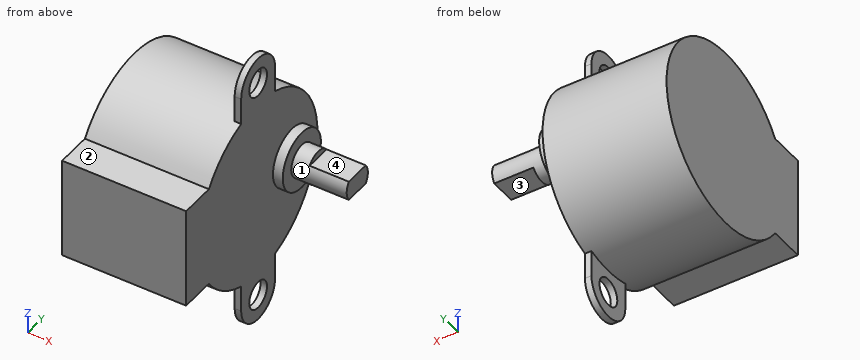
Autodesk Inventor part; units mm, degrees
ref_plane "YZ Plane" through (0, 0, 0) normal (1, 0, 0) x (0, 1, 0)
ref_plane "XZ Plane" through (0, 0, 0) normal (0, 1, 0) x (-1, 0, 0)
ref_plane "XY Plane" through (0, 0, 0) normal (0, 0, 1) x (1, 0, 0)
sketch "Boceto1" plane through (0, 0, 0) normal (1, 0, 0) x (0, 1, 0)
  circle A0 centre (0, 0) radius 14
  dimension "d0" = 28
extrude "Extrusión1" add sketch "Boceto1" along normal blind 19
sketch "Boceto2" plane through (19, 0, 0) normal (1, 0, 0) x (0, 0, -1)
  line L0 (0, 0) -> (0, 8)
  circle A0 centre (0, 8) radius 4.5
  dimension "d3" = 8
  dimension "d4" = 9
extrude "Extrusión2" add sketch "Boceto2" along normal blind 1.5
sketch "Boceto3" plane through (20.5, 8, 0) normal (1, 0, 0) x (0, 0, -1)
  circle A0 centre (0, 0) radius 2.5
  point P0 (0, -8)
  dimension "d7" = 5
extrude "Extrusión3" add sketch "Boceto3" along normal blind 2.5
sketch "Boceto4" plane through (23, 8, 0) normal (1, 0, 0) x (0, 0, -1)
  line L0 (0, 0) -> (-1.5, 0)
  line L1 (-1.5, 0) -> (-1.5, 3)
  line L2 (-1.5, 3) -> (-1.5, -3)
  line L3 (-1.5, -3) -> (1.5, -3)
  line L4 (1.5, -3) -> (1.5, 2.8642)
  circle A0 centre (0, 0) radius 2.5
  point P0 (0, -8)
  point P1 (1.5, 2)
  point P2 (-1.5, 2)
  point P3 (-1.5, -2)
  point P4 (1.5, -2)
  dimension "d10" = 1.5
  dimension "d11" = 3
extrude "Extrusión4" add sketch "Boceto4" along normal blind 6 contours L1 A0 L4 L2
sketch "Boceto5" plane through (19, 0, 0) normal (1, 0, 0) x (0, 0, -1)
  line L0 (0, 0) -> (17.5, 0)
  circle A0 centre (17.5, 0) radius 2.1
  arc A1 (17.5, -4) -> (17.5, 4) centre (17.5, 0) ccw
  line L1 (17.5, 4) -> (-17.5, 4)
  line L2 (0, 0) -> (0, 18)
  line L3 (-15.4, 0) -> (-17.5, 0)
  circle A2 centre (-17.5, 0) radius 2.1
  arc A3 (-17.5, 4) -> (-17.5, -4) centre (-17.5, 0) ccw
  line L4 (17.5, -4) -> (-17.5, -4)
  dimension "d18" = 4.2
  dimension "d14" = 17.5
  dimension "d15" = 4.2
  dimension "d16" = 8
  dimension "d17" = 17.5
  dimension "d19" = 8
extrude "Extrusión5" add sketch "Boceto5" against normal blind 1
sketch "Boceto6" plane through (19, 0, 0) normal (1, 0, 0) x (0, 0, -1)
  line L0 (0, 0) -> (0, -17)
  line L1 (0, -17) -> (7.8, -17)
  line L2 (0, -17) -> (-7.8, -17)
  line L3 (-7.8, -17) -> (7.8, -17)
  line L4 (7.8, -17) -> (7.8, -6)
  line L5 (7.8, -6) -> (-7.8, -6)
  line L6 (-7.8, -6) -> (-7.8, -17)
  dimension "d22" = 17
  dimension "d23" = 7.8
  dimension "d25" = 7.8
extrude "Extrusión6" add sketch "Boceto6" against normal blind 19
properties part number "MOTOR"
Design review of the part built by this model. Coordinates are the model's own, in mm. Face numbers are marked on the shaded views. A direction names the side the tool comes from. Give positions to 0.01 mm unless a question says otherwise; leave off trailing zeros. Write each loop counter-clockwise with the first axis right and the second up, starting at its lowest first coordinate (ties: lowest second). Pieces come first, ordered by that corner, then holes. Notation, with made-up numbers: M -10.5,11.5 L 46.5,11.5 A21 cw 46.5,16.5 Z; hole C 10,2.5 d2. An arc over 180 degrees is marked long. Return JSON: item names as keys, results as strings. Group by question number.
Item 1: Tool access review of the marked faces 1, 2, 3 and 4: name each direction out of +Z, -Z, +X, -X, +Y, -Y from which nothing blocks a thin tool from reaching the whole face with its end or side.
Item 2: Take a section at B-B (z = 0). Give the boundary of the cut face in (x, y).
Item 3: Take a section at A-A (y = 0). Give the boundary of the cut face in (x, z), plus the area to 3 significant figures.
Item 4: Take a section at C-C (x = 17.25). Give the boundary of the cut face in (y, z), plus the area to 3 significant figures.
Item 5: Wall thickness on line 1 along Y through (x, z) = (18.2, 17.5); line 2 along X through (y, z) = (-3, 10); line 3 along Z through (x, y) = (1.5, -13.5): over which ranges is each line inside the solid? List them lowest first.
Item 6: Take a section at D-D (z = -16). Give the boundary of the cut face in (x, y).
Item 7: Clearance check with flat-ended pins moving along their axes: pin 1 Ø6 at (x, y) = (13, 8.5) entering from +Z; pin 2 Ø6.5 at (y, z) = (0, -17.5) entering from +X; pin 3 Ø5 at (x, y) = (14, -11) entering from -Z; pin 4 Ø1.1 at (y, z) = (7.5, -2) entering from +X. State where each tip first meets the part, or that it passes through.
Return value:
{
 "1": {"face 1": "+X", "face 2": "+Z, +X, -X, -Y", "face 3": "-Z, +X, +Y, -Y", "face 4": "+Z, +X, +Y, -Y"},
 "2": {"outline": "M 0,-17 L 19,-17 L 19,3.5 L 20.5,3.5 L 20.5,5.5 L 29,5.5 L 29,10.5 L 20.5,10.5 L 20.5,12.5 L 19,12.5 L 19,14 L 0,14 Z"},
 "3": {"outline": "M 0,-14 L 18,-14 L 18,-15.4 L 19,-15.4 L 19,15.4 L 18,15.4 L 18,14 L 0,14 Z; M 18,-21.5 L 19,-21.5 L 19,-19.6 L 18,-19.6 Z; M 18,19.6 L 19,19.6 L 19,21.5 L 18,21.5 Z", "area": "539 mm2"},
 "4": {"outline": "M -17,-7.8 L -11.63,-7.8 A14 ccw long -11.63,7.8 L -17,7.8 Z", "area": "674 mm2"},
 "5": {"line 1": "y = -4 to -2.1, 2.1 to 4", "line 2": "x = 0 to 19", "line 3": "z = -7.8 to 7.8"},
 "6": {"outline": "M 18,-4 L 19,-4 L 19,-1.47 L 18,-1.47 Z; M 18,1.47 L 19,1.47 L 19,4 L 18,4 Z"},
 "7": {"pin 1": "stops at z = 12.87", "pin 2": "stops at x = 19", "pin 3": "stops at z = -11.12", "pin 4": "stops at x = 29"}
}
